Geometry: final body of the model. Coordinates: model frame, mm. A direction names the side the tool comes from. Coordinates: 2 decimals unless noted, no trailing zeros. Write each loop counter-clockwise with the first axis right and the second up, starting at its lowest first coordinate (ties: lowest second). Pieces come first, ordered by that corner, then holes.
from build123d import *

# Parameters (mm, degrees)
SKETCH1_R           = 11
SKETCH1_R_2         = 4
BOSS_EXTRUDE1_DEPTH = 3.5
SKETCH2_R           = 4
CUT_EXTRUDE3_DEPTH  = 6.4
CIRPATTERN1_COUNT   = 6
SKETCH3_R           = 4.05
BOSS_EXTRUDE2_DEPTH = 6


with BuildPart() as part:
    # Sketch1 → Boss-Extrude1 (new body, symmetric)
    with BuildSketch(Plane.XY):
        Circle(SKETCH1_R)
        Circle(SKETCH1_R_2, mode=Mode.SUBTRACT)
    extrude(amount=BOSS_EXTRUDE1_DEPTH, both=True)

    # Sketch2 → Cut-Extrude3 (cut)
    with BuildSketch(Plane(origin=(-11, -17.193061184, 0), x_dir=(0, -1, 0), z_dir=(1, 0, 0))):
        with Locations((-17.193061184, 0)):
            Circle(SKETCH2_R)
    cut_extrude3 = extrude(amount=CUT_EXTRUDE3_DEPTH, mode=Mode.SUBTRACT)

    # CirPattern1: Cut-Extrude3 ×6 about axis
    cirpattern1_axis = Axis((0, 0, 0), (0, 0, 1))
    for i in range(1, CIRPATTERN1_COUNT):
        add(cut_extrude3.rotate(cirpattern1_axis, i * 360 / CIRPATTERN1_COUNT), mode=Mode.SUBTRACT)

    # Sketch3 → Boss-Extrude2 (add)
    with BuildSketch(Plane(origin=(-4.6, 0, 0), x_dir=(0, -1, 0), z_dir=(-1, 0, 0))):
        Circle(SKETCH3_R)
    extrude(amount=BOSS_EXTRUDE2_DEPTH)


solid = part.part
Item 1: Set-up query: faces 1 (the flat face through (-4.6, 3, 0)), 2 (the flat face through (2.27, -4, -0.05)), 3 (the cylindrical face through (-10.45, -4.05, -0.04)). Return all of +Z, -Z, +X, -X, +Y, -Y with unobstructed straight access to the full face (end or side cutting, diameter ignored); none if empty.
Derived:
face 1: +Y
face 2: none
face 3: -X, -Y
Item 2: Material intervals for probe 1 along Y at (x, z) = (1.75, -3); probe 2 along X at (y, z) = (3.25, 0.75); probe 3 along Z at (x, y) = (5.75, 3.75), sorted ascending.
Derived:
probe 1: y = -10.86 to -8.32, -4.3 to -3.6, 3.6 to 4.3, 8.32 to 10.86
probe 2: x = -10.6 to -4.6, -3.57 to -2.33, 2.33 to 3.57
probe 3: z = -3.5 to -2.52, 2.52 to 3.5
Item 3: Section A-A, the plane y = 0. Output: boundary loops of the cut face in (x, z).
Derived:
outline: (-10.6, -4.05) - (-4.6, -4.05) - (-4.6, -3.5) - (-4, -3.5) - (-4, 3.5) - (-4.6, 3.5) - (-4.6, 4.05) - (-10.6, 4.05) - close; (4, -3.5) - (4.6, -3.5) - (4.6, 3.5) - (4, 3.5) - close
Item 4: Pin query (flat end, axial travel): pin 1 (1 mm diameter, centred on y = -2, z = -1.5, fed in from +X); pin 2 (11 mm diameter, centred on x = -1, y = -3, fed in from +Z); pin 3 (11 mm diameter, centred on x = 4.5, y = -3, fed in from -Z); pin 4 (1 mm diameter, centred on x = 3.5, z = -3, fed in from -Y). Return the tip coordinate at first contact, or that it passes through.
Derived:
pin 1: stops at x = 4.6
pin 2: stops at z = 4.05
pin 3: stops at z = -3.5
pin 4: stops at y = -10.58
Item 5: Pull-direction query (Z, two-part tool) for faces 4 (the cylindrical face through (-10.45, 4.05, 0.04)), 5 (the flat face through (-2.27, 4, -0.05)); classes: released by +Z, released by -Z, zero draft, split by the parting line, or undercut.
Derived:
face 4: split by the parting line
face 5: undercut
Item 6: Section B-B, the plane z = 1. State how many separate pieces and enclosed holes the cut face has, plus the area to 3 significant figures.
Derived:
separate pieces: 5
enclosed holes: 1
area: 105 mm2
